Could you check a few things on this drawing? It's one solid part, dimensions in mm from its lowest x, y, z. A direction names the side the tool comes from. Coordinates: 2 decimals unless noted, no trailing zeros. Order: outer loops, then holes, each group sorted by start corner. A loop starts at its lowest first (then second) coordinate and runs counter-clockwise, first axis right, second up.
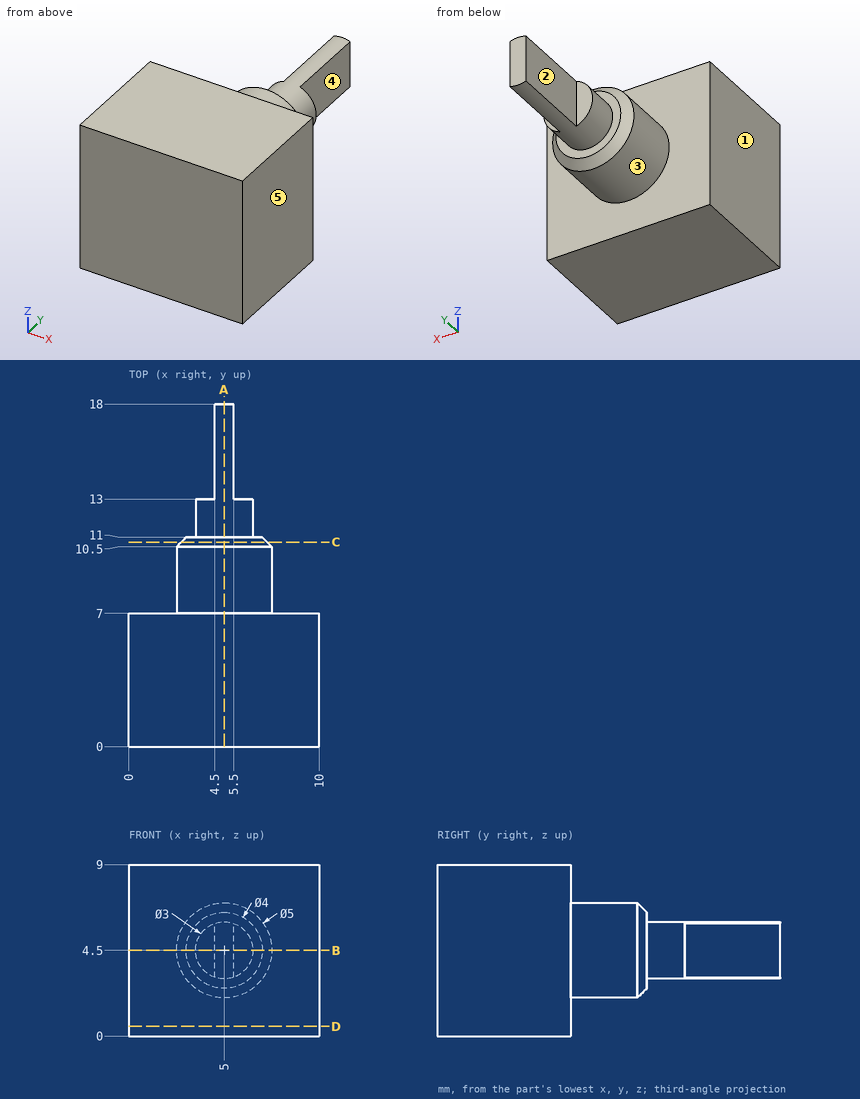
1. Imagine slicing it at D-D on z = 0.5. Please give me the cut outline in (x, y).
Completed:
outline: (0, 0) - (10, 0) - (10, 7) - (0, 7) - close
2. Imagine slicing it at A-A on x = 5. Please give me the cut outline in (y, z).
Completed:
outline: (0, 0) - (7, 0) - (7, 2) - (10.5, 2) - (11, 2.5) - (11, 3) - (18, 3) - (18, 6) - (11, 6) - (11, 6.5) - (10.5, 7) - (7, 7) - (7, 9) - (0, 9) - close
3. On a 3-axis mill with a long thin cutter (end or side, diameter ignored), from which of +Z, -Z, +X, -X, +Y, -Y can I reach the whole of each face in a straight line? I mean the marked faces 1, 2, 3, 4 and 5. Say none if no direction works.
Completed:
face 1: +Z, -Z, -X, +Y, -Y
face 2: +Z, -Z, -X, +Y
face 3: +Y
face 4: +Z, -Z, +X, +Y
face 5: +Z, -Z, +X, +Y, -Y
4. Please list where these lines run through material, in increasing order: probe 1 along X at (y, z) = (9.25, 6.5); probe 2 along Y at (x, z) = (2.75, 0.5); probe 3 along X at (y, z) = (7.25, 3).
Completed:
probe 1: x = 3.5 to 6.5
probe 2: y = 0 to 7
probe 3: x = 3 to 7
5. I'm going to push flat-ended pins straight in: pin 1 (0.8 mm diameter, centred on y = 16, z = 5, fed in from -X); pin 2 (3 mm diameter, centred on y = 12, z = 3, fed in from -X); pin 3 (1 mm diameter, centred on y = 10.5, z = 5.5, fed in from -X). Where does each tip first touch, or does it pass through?
Completed:
pin 1: stops at x = 4.5
pin 2: stops at x = 2.8
pin 3: stops at x = 2.55
6. Imagine slicing it at B-B on z = 4.5. Please give me the cut outline in (x, y).
Completed:
outline: (0, 0) - (10, 0) - (10, 7) - (7.5, 7) - (7.5, 10.5) - (7, 11) - (6.5, 11) - (6.5, 13) - (5.5, 13) - (5.5, 18) - (4.5, 18) - (4.5, 13) - (3.5, 13) - (3.5, 11) - (3, 11) - (2.5, 10.5) - (2.5, 7) - (0, 7) - close
7. Imagine slicing it at C-C on y = 10.75. Please give me the cut outline in (x, z).
Completed:
outline: circle Ø4.5 at (5, 4.5)
